Read the model definition and answer for the solid it produces. Units are mm, in the model's axes. A direction names the side the tool comes from. Coordinates: 2 decimals unless noted, no trailing zeros. Order: outer loops, then holes, each group sorted by start corner. A loop starts at its lowest first (then second) coordinate and runs counter-clockwise, first axis right, second up. Notation, with made-up numbers: M 83,-4.75 L 105,-4.75 A14 cw 105,14.25 Z; hole C 7.5,19.5 d3. An arc over 180 degrees is marked long. One line per question, with ' | ' between items. Start each with the question number.
1) Find section D-D, the plane x = -12. Write down the section's boundary in (y, z).
2) Find section A-A, the plane x = -17.5. Count the separate pieces of the cut face and the enclosed holes in it, plus the area to 3 significant figures.
3) Given P1, Ø2, axis at y = 18, z = 3, coming from the +X side; P2, Ø1.3, axis at x = 7, z = 0.5, coming from the +Y side; P3, Ø1, axis at x = -12, z = 3, coming from the -Y side, each flat-ended and moving along its own axis, determine where each tip first touches the part or whether it passes through.
4) Consider probe 1 along Y at (x, z) = (17.5, 1.2) (3 decimals); probe 2 along X at (y, z) = (11, 0.45); probe 3 along Y at (x, z) = (-15, 2.5). Determine where each line is inside the solid, lowest interval first.
5) A tool of negligible diameter and unlimited length cuts with its end or side. For faces 1 (the face through (-12.878, 20.384, 4.614)), 2 (the face through (13, 16.55, 1)), from which of +Z, -Z, +X, -X, +Y, -Y can it reach the whole face along a straight path? Write none if from no direction.
6) The mould has two halves that part along Z. Classify faces 3 (the face through (0, 10, 0)), 4 (the face through (-12.878, 19.794, 2.402)), 5 (the face through (20.497, 8.407, 0.783)): +Z half, -Z half, draft (parallel to the pull), parting line (faces both ways), or undercut.
7) Find section B-B, the plane z = 2.5. Write down the section's boundary in (x, y).
from build123d import *

# Parameters (mm, degrees)
SKETCH1_W                   = 50.8
SKETCH1_H                   = 19.05
BOSS_EXTRUDE1_DEPTH         = 1.5875
SKETCH2_R                   = 2.5
SKETCH2_R_2                 = 0.75
BOSS_EXTRUDE2_DEPTH         = 25.4
CUT_EXTRUDE2_DEPTH          = 25.4
F_6_0_MM_DOWEL_HOLES1_D     = 6
F_6_0_MM_DOWEL_HOLES1_DEPTH = 30
F_6_0_MM_DOWEL_HOLES1_TIP   = 1.802581857


with BuildPart() as part:
    # Sketch1 → Boss-Extrude1 (new body)
    with BuildSketch(Plane.XY):
        with Locations((0, 9.525)):
            Rectangle(SKETCH1_W, SKETCH1_H)
    extrude(amount=BOSS_EXTRUDE1_DEPTH)

    # Sketch2 → Boss-Extrude2 (add)
    with BuildSketch(Plane.ZY.offset(25.4)):
        with Locations((2.5, 19.05)):
            Circle(SKETCH2_R)
        with Locations((2.5, 19.05)):
            Circle(SKETCH2_R_2, mode=Mode.SUBTRACT)
    extrude(amount=-BOSS_EXTRUDE2_DEPTH)

    # Sketch3 → Cut-Extrude2 (cut)
    with BuildSketch(Plane(origin=(0, 0, 0), x_dir=(0, 0, -1), z_dir=(1, 0, 0))):
        with BuildLine():
            Line((-2.5, 16.55), (0, 16.55))
            Line((0, 16.55), (0, 19.05))
            ThreePointArc((0, 19.05), (-4.267766953, 20.817766953), (-2.5, 16.55))
        make_face()
    extrude(amount=CUT_EXTRUDE2_DEPTH, mode=Mode.SUBTRACT)

    # Ø6.0 mm Dowel Holes1
    with Locations(Plane.XY.offset(1.5875)):
        with Locations((-17.5, 8.275), (17.5, 8.275)):
            Hole(F_6_0_MM_DOWEL_HOLES1_D / 2, depth=F_6_0_MM_DOWEL_HOLES1_DEPTH)
            with Locations((0, 0, -(F_6_0_MM_DOWEL_HOLES1_DEPTH + F_6_0_MM_DOWEL_HOLES1_TIP / 2))):  # 118° drill point
                Cone(0, F_6_0_MM_DOWEL_HOLES1_D / 2, F_6_0_MM_DOWEL_HOLES1_TIP, mode=Mode.SUBTRACT)


solid = part.part
Report:
1) outline: M 0,0 L 19.05,0 A2.5 ccw long 16.72,1.59 L 0,1.59 Z; hole C 19.05,2.5 d1.5
2) separate pieces: 2 | enclosed holes: 1 | area: 35.9 mm^2
3) P1: stops at x = 0 | P2: stops at y = 16.55 | P3: stops at y = 16.55
4) probe 1: y = 0 to 5.275, 11.275 to 16.55 | probe 2: x = -25.4 to -18.75, -16.25 to 16.25, 18.75 to 25.4 | probe 3: y = 16.55 to 18.3, 19.8 to 21.55
5) face 1: +X, -X | face 2: +Z, -Z, +X, +Y
6) face 3: -Z half | face 4: undercut | face 5: draft
7) outline: M -25.4,16.55 L 0,16.55 L 0,18.3 L -25.4,18.3 Z; M -25.4,19.8 L 0,19.8 L 0,21.55 L -25.4,21.55 Z
